```python
from build123d import *

# Parameters (mm, degrees)
SKETCH1_R           = 15.875
BASE_EXTRUDE_DEPTH  = 50.8
SKETCH2_R           = 19.05
BOSS_EXTRUDE1_DEPTH = 254
SKETCH3_R           = 15.875
BOSS_EXTRUDE2_DEPTH = 76.2
FILLET1_R           = 25.4
FILLET2_R           = 38.1
CUT_EXTRUDE1_DEPTH  = 38.1
CUT_EXTRUDE2_DEPTH  = 38.1


with BuildPart() as part:
    # Sketch1 → Base-Extrude (new body)
    with BuildSketch(Plane(origin=(0, 0, 0), x_dir=(0, 0, -1), z_dir=(1, 0, 0))):
        Circle(SKETCH1_R)
    extrude(amount=BASE_EXTRUDE_DEPTH)

    # Sketch2 → Boss-Extrude1 (add)
    with BuildSketch(Plane(origin=(50.8, 0, 0), x_dir=(0, 0, -1), z_dir=(1, 0, 0))):
        Circle(SKETCH2_R)
    extrude(amount=BOSS_EXTRUDE1_DEPTH)

    # Sketch3 → Boss-Extrude2 (add)
    with BuildSketch(Plane(origin=(304.8, 0, 0), x_dir=(0, 0, -1), z_dir=(1, 0, 0))):
        Circle(SKETCH3_R)
    extrude(amount=BOSS_EXTRUDE2_DEPTH)

    # Fillet1
    # the kernel refuses this fillet: 25.4 mm, written as the material it adds along each edge
    with BuildSketch(Plane(origin=(304.8, 0, 0), x_dir=(0, 0, -1), z_dir=(0, -1, 0))) as fillet1_piece_1:
        with BuildLine():
            CenterArc((41.275, 12.296722124), FILLET1_R, 180, 28.955024372)
            Line((15.875, 12.296722124), (15.367, 12.296722124))
            Line((15.367, 12.296722124), (15.367, 0))
            Line((15.367, 0), (15.875, -0.508))
            ThreePointArc((15.875, -0.508), (17.4625, -0.508), (18.6055, -0.245934442))
            Line((18.6055, -0.245934442), (19.05, 0))
        make_face()
    revolve(axis=Axis((304.8, 0, 0), (1, 0, 0)))

    # Fillet2
    # the kernel refuses this fillet: 38.1 mm, written as the material it adds along each edge
    with BuildSketch(Plane(origin=(50.8, 0, 0), x_dir=(0, 0, -1), z_dir=(0, -1, 0))) as fillet2_piece_1:
        with BuildLine():
            CenterArc((53.975, -15.226765087), FILLET2_R, 156.443535691, 23.556464309)
            Line((15.875, -15.226765087), (15.113, -15.226765087))
            Line((15.113, -15.226765087), (15.113, 0))
            Line((15.113, 0), (15.875, 0.762))
            ThreePointArc((15.875, 0.762), (17.4625, 0.762), (18.3515, 0.304535302))
            Line((18.3515, 0.304535302), (19.05, 0))
        make_face()
    revolve(axis=Axis((50.8, 0, 0), (1, 0, 0)))

    # Sketch4 → Cut-Extrude1 (cut, symmetric)
    with BuildSketch(Plane.XY):
        with BuildLine():
            Line((341.301045638, 6.648208461), (381, 3.175))
            Line((381, 3.175), (381, 15.875))
            Line((381, 15.875), (323.85, 15.875))
            ThreePointArc((323.85, 15.875), (331.642512816, 9.496960468), (341.301045638, 6.648208461))
        make_face()
    cut_extrude1 = extrude(amount=CUT_EXTRUDE1_DEPTH, both=True, mode=Mode.SUBTRACT)

    # Mirror1: Cut-Extrude1 across plane
    add(cut_extrude1.mirror(Plane.ZX), mode=Mode.SUBTRACT)

    # Sketch5 → Cut-Extrude2 (cut, symmetric)
    with BuildSketch(Plane(origin=(0, 0, 0), x_dir=(1, 0, 0), z_dir=(0, 1, 0))):
        Polygon((361.95, 15.875), (381, 4.876477372), (381, 15.875), align=None)
    cut_extrude2 = extrude(amount=CUT_EXTRUDE2_DEPTH, both=True, mode=Mode.SUBTRACT)

    # Mirror2: Cut-Extrude2 across plane
    add(cut_extrude2.mirror(Plane.XY), mode=Mode.SUBTRACT)


solid = part.part
```
Verification items for the finished model (mm, model axes). A direction names the side the tool comes from. Round coordinates to 2 decimals unless told otherwise and drop trailing zeros. Order: outer loops, then holes, each group sorted by start corner. A loop starts at its lowest first (then second) coordinate and runs counter-clockwise, first axis right, second up.
1) Draft check along Z on faces 1 (the cylindrical face through (176.02, -11.59, 15.12)), 2 (the flat face through (371.342, 0.066, 10.453)), 3 (the flat face through (356.46, 5.32, 0.21)), 4 (the flat face through (371.342, 0.066, -10.453)). Enter one of: +Z half, -Z half, draft (parallel to the pull), parting line (faces both ways), or undercut.
Geometry says:
face 1: parting line
face 2: +Z half
face 3: draft
face 4: -Z half
2) Cross-section at B-B, the plane z = 0. Record the cut outline in (x, y) (3 decimals), plus the area to 3 significant figures.
Geometry says:
outline: (0, -15.875) - (35.573, -15.875) arc R38.1 cw to (50.8, -19.05) - (304.8, -19.05) arc R25.4 cw to (317.097, -15.875) - (323.85, -15.875) arc R25.4 cw to (341.301, -6.648) - (381, -3.175) - (381, 3.175) - (341.301, 6.648) arc R25.4 cw to (323.85, 15.875) - (317.097, 15.875) arc R25.4 cw to (304.8, 19.05) - (50.8, 19.05) arc R38.1 cw to (35.573, 15.875) - (0, 15.875) - close
area: 12,700 mm2
3) Depth check by flat-ended pin: pin 1 (1.5 mm diameter, centred on x = 274, z = -14.5, fed in from -Y); pin 2 (10 mm diameter, centred on x = 323, z = -4.5, fed in from +Y) (3 decimals); pin 3 (4 mm diameter, centred on x = 336, y = -4, fed in from -Z); pin 4 (12 mm diameter, centred on y = -6, z = -3, fed in from -X). Enter the tip coordinate at first touch or a pass-through.
Geometry says:
pin 1: stops at y = -13.18
pin 2: stops at y = 15.875
pin 3: stops at z = -15.75
pin 4: stops at x = 0
4) Tool access check on faces 5 (the cylindrical face through (17.538, -15.497, 3.441)), 6 (the cylindrical face through (333.55, 8.59, 0.2)), 7 (the cylindrical face through (334.7, 4.77, -15.14)). Record the directions out of +Z, -Z, +X, -X, +Y, -Y that give a thin tool (end or side, any length) a straight path to the whole face; none if there is none.
Geometry says:
face 5: -X
face 6: +Z, -Z, +X, +Y
face 7: +X
5) Cross-section at A-A, the plane y = 0. Record the cut outline in (x, z) (3 decimals), plus the area to 3 significant figures.
Geometry says:
outline: (0, -15.875) - (35.573, -15.875) arc R38.1 cw to (50.8, -19.05) - (304.8, -19.05) arc R25.4 cw to (317.097, -15.875) - (361.95, -15.875) - (381, -4.876) - (381, 4.876) - (361.95, 15.875) - (317.097, 15.875) arc R25.4 cw to (304.8, 19.05) - (50.8, 19.05) arc R38.1 cw to (35.573, 15.875) - (0, 15.875) - close
area: 13,600 mm2
6) Cross-section at D-D, the plane x = 29.5. Record the cut outline in (y, z) (3 decimals), plus the area to 3 significant figures.
Geometry says:
outline: circle Ø31.75 at (0, 0)
area: 792 mm2
7) Cross-section at C-C, the plane x = 108. Record the cut outline in (y, z).
Geometry says:
outline: circle Ø38.1 at (0, 0)
8) Material ranges on line 1 (Z direction, x = 268.5, y = -0.5); line 2 (Y direction, x = 183.5, z = 10.5); line 3 (Y direction, x = 59, z = 12.5), recorded low to high.
Geometry says:
line 1: z = -19.04 to 19.04
line 2: y = -15.9 to 15.9
line 3: y = -14.38 to 14.38
